The model under review builds one solid part; all positions refer to its coordinate system, in mm. A direction names the side the tool comes from. Give positions to 0.01 mm unless a question says otherwise; leave off trailing zeros. Write each loop counter-clockwise with the first axis right and the second up, starting at its lowest first coordinate (ties: lowest second). Pieces come first, ordered by that corner, then holes. Notation, with made-up numbers: (56, -21.75) -> (106, -21.75) arc R16 cw to (106, -10.75) -> close; hole circle Ø8 at (-9.5, 53.5). An arc over 180 degrees is marked (long way). Use CSV: the item, a comma, the result in double quotes.
```python
from build123d import *

# Parameters (mm, degrees)
F0_W     = 22.225
F0_H     = 22.225
F0_W_2   = 25.4
F0_H_2   = 25.4
F0_H_3   = 3.175
F0_W_3   = 3.175
F1_DEPTH = 3.175


with BuildPart() as f1:
    # F0 (on Top) → F1 (new body)
    with BuildSketch(Plane.XY):
        with Locations((-49.2125, 49.2125)):
            Rectangle(F0_W, F0_H)
        with Locations((-25.4, 49.2125)):
            Rectangle(F0_W_2, F0_H)
        with Locations((25.4, 49.2125)):
            Rectangle(F0_W_2, F0_H)
        with Locations((49.2125, 49.2125)):
            Rectangle(F0_W, F0_H)
        with Locations((49.2125, 25.4)):
            Rectangle(F0_W, F0_H_2)
        with Locations((25.4, 25.4)):
            Rectangle(F0_W_2, F0_H_2)
        with Locations((0, 25.4)):
            Rectangle(F0_W_2, F0_H_2)
        with Locations((-25.4, 25.4)):
            Rectangle(F0_W_2, F0_H_2)
        with Locations((-49.2125, 25.4)):
            Rectangle(F0_W, F0_H_2)
        with Locations((-49.2125, 0)):
            Rectangle(F0_W, F0_H_2)
        with Locations((-25.4, 0)):
            Rectangle(F0_W_2, F0_H_2)
        Rectangle(F0_W_2, F0_H_2)
        with Locations((25.4, 0)):
            Rectangle(F0_W_2, F0_H_2)
        with Locations((49.2125, 0)):
            Rectangle(F0_W, F0_H_2)
        with Locations((49.2125, -25.4)):
            Rectangle(F0_W, F0_H_2)
        with Locations((25.4, -25.4)):
            Rectangle(F0_W_2, F0_H_2)
        with Locations((0, -25.4)):
            Rectangle(F0_W_2, F0_H_2)
        with Locations((-25.4, -25.4)):
            Rectangle(F0_W_2, F0_H_2)
        with Locations((-49.2125, -25.4)):
            Rectangle(F0_W, F0_H_2)
        with Locations((-49.2125, -49.2125)):
            Rectangle(F0_W, F0_H)
        with Locations((-25.4, -49.2125)):
            Rectangle(F0_W_2, F0_H)
        with Locations((25.4, -49.2125)):
            Rectangle(F0_W_2, F0_H)
        with Locations((49.2125, -49.2125)):
            Rectangle(F0_W, F0_H)
        with Locations((0, 49.2125)):
            Rectangle(F0_W_2, F0_H)
        with Locations((0, -49.2125)):
            Rectangle(F0_W_2, F0_H)
        with Locations((-25.4, -61.9125)):
            Rectangle(F0_W_2, F0_H_3)
        with Locations((-61.9125, -25.4)):
            Rectangle(F0_W_3, F0_H_2)
        with Locations((-61.9125, 25.4)):
            Rectangle(F0_W_3, F0_H_2)
        with Locations((-25.4, 61.9125)):
            Rectangle(F0_W_2, F0_H_3)
        with Locations((25.4, 61.9125)):
            Rectangle(F0_W_2, F0_H_3)
        with Locations((61.9125, 25.4)):
            Rectangle(F0_W_3, F0_H_2)
        with Locations((61.9125, -25.4)):
            Rectangle(F0_W_3, F0_H_2)
        with Locations((25.4, -61.9125)):
            Rectangle(F0_W_2, F0_H_3)
    extrude(amount=F1_DEPTH)


solid = f1.part
```
Q1. To check wall thickness, follow probe 1 along X at (y, z) = (9, 0.65) (3 decimals). State the ranges of the line that lie inside material, in increasing order.
Derived:
probe 1,"x = -60.325 to 60.325"
Q2. Machinability: for faces 5 (the flat face through (0, 60.325, 2)), 6 (the flat face through (49, 60.325, 2)), 7 (the flat face through (-62, -12.7, 2)), 8 (the flat face through (-12.7, -62, 2)), which of the approach directions +Z, -Z, +X, -X, +Y, -Y give a long, thin tool a straight path to every point of the face, cutting with its end or side? Answer none if there is none.
Derived:
face 5,"+Z, -Z, +Y"
face 6,"+Z, -Z, +X, +Y"
face 7,"+Z, -Z, -X"
face 8,"+Z, -Z, -Y"
Q3. The part is to be moulded in two halves that separate along Y. For faces 1 (the flat face through (-62, -38.1, 2)), 2 (the flat face through (62, 12.7, 2)), 3 (the flat face through (62, -12.7, 2)), 4 (the flat face through (62, 38.1, 2)), say which applies: pulls with the +Y half, pulls with the -Y half, needs draft (parallel to the pull), parting line crosses it, or undercut.
Derived:
face 1,"pulls with the -Y half"
face 2,"undercut"
face 3,"undercut"
face 4,"pulls with the +Y half"
Q4. Insertion check: pin 1 (1.6 mm diameter, centred on y = 54, z = 1.5, fed in from -X) (3 decimals); pin 2 (1 mm diameter, centred on y = 62.5, z = 1.5, fed in from -X); pin 3 (1.6 mm diameter, centred on x = 62, z = 1.5, fed in from +Y). Each pin has a flat end and moves straight along its axis. Give the tip position at first contact, or say it passes through.
Derived:
pin 1,"stops at x = -60.325"
pin 2,"stops at x = -38.1"
pin 3,"stops at y = 38.1"
Q5. Consider section A-A (x = -8). Write out the cut boundary in (y, z) (3 decimals).
Derived:
outline,"(-60.325, 0) -> (60.325, 0) -> (60.325, 3.175) -> (-60.325, 3.175) -> close"
